Build history of the part. All positions in model axes, mm. A direction names the side the tool comes from. Round coordinates to 2 decimals unless told otherwise and drop trailing zeros. Order: outer loops, then holes, each group sorted by start corner. A loop starts at its lowest first (then second) coordinate and runs counter-clockwise, first axis right, second up. Notation, with made-up numbers: M -34,5 L 9,5 A12 cw 9,15 Z; hole C -5,0.5 d1. An arc over 180 degrees is marked long. One line per item, written item: value. Start each with the question number.
Item 1: Band-saw the part on A-A, the plane x = -9. Write the cut outline in (y, z).
Item 2: Probe L1, parallel to Y at x = 15, z = 0.3; L2, parallel to Y at x = 16.5, z = 0.4. List the from-to ranges inside material, lowest first.
Item 3: Two-plate mould, pull along X, no slides. Class faces 3 (the cylindrical face through (17.1, 10.86, 0.69)), 4 (the flat face through (17, 75, 1)), 5 (the flat face through (10, 74, 1)): +X half, -X half, draft (parallel to the pull), parting line (faces both ways), or undercut.
Item 4: Tool access for faces 1 (the flat face through (-7, 75, 1)), 2 (the flat face through (15, 73, 1)): list every direction of +Z, -Z, +X, -X, +Y, -Y with a clear straight run to the whole face (end or side of a thin tool).
```python
from build123d import *

# Parameters (mm, degrees)
F1_DEPTH = 1.4


with BuildPart() as f1:
    # F0 (on Top) → F1 (new body)
    with BuildSketch(Plane.XY):
        with BuildLine():
            Line((-18, 75), (-20, 75))
            Line((-20, 75), (-20, 73))
            Line((-20, 73), (-20, 13))
            ThreePointArc((-20, 13), (-19.12132, 10.87868), (-17, 10))
            Line((-17, 10), (-13, 10))
            Line((-13, 10), (13, 10))
            Line((13, 10), (15, 10))
            ThreePointArc((15, 10), (17.12132, 10.87868), (18, 13))
            Line((18, 13), (18, 73))
            Line((18, 73), (18, 75))
            Line((18, 75), (16, 75))
            Line((16, 75), (16, 73))
            Line((16, 73), (14, 73))
            Line((14, 73), (14, 75))
            Line((14, 75), (12, 75))
            Line((12, 75), (12, 73))
            Line((12, 73), (10, 73))
            Line((10, 73), (10, 75))
            Line((10, 75), (8, 75))
            Line((8, 75), (8, 73))
            Line((8, 73), (6, 73))
            Line((6, 73), (6, 75))
            Line((6, 75), (4, 75))
            Line((4, 75), (4, 73))
            Line((4, 73), (2, 73))
            Line((2, 73), (2, 75))
            Line((2, 75), (0, 75))
            Line((0, 75), (0, 73))
            Line((0, 73), (-2, 73))
            Line((-2, 73), (-2, 75))
            Line((-2, 75), (-4, 75))
            Line((-4, 75), (-4, 73))
            Line((-4, 73), (-6, 73))
            Line((-6, 73), (-6, 75))
            Line((-6, 75), (-8, 75))
            Line((-8, 75), (-8, 73))
            Line((-8, 73), (-10, 73))
            Line((-10, 73), (-10, 75))
            Line((-10, 75), (-12, 75))
            Line((-12, 75), (-12, 73))
            Line((-12, 73), (-14, 73))
            Line((-14, 73), (-14, 75))
            Line((-14, 75), (-16, 75))
            Line((-16, 75), (-16, 73))
            Line((-16, 73), (-18, 73))
            Line((-18, 73), (-18, 75))
        make_face()
    extrude(amount=F1_DEPTH)


solid = f1.part
```
Output:
1. outline: M 10,0 L 73,0 L 73,1.4 L 10,1.4 Z
2. L1: y = 10 to 73
2. L2: y = 10.4 to 75
3. face 3: +X half
3. face 4: draft
3. face 5: undercut
4. face 1: +Z, -Z, +X, -X, +Y
4. face 2: +Z, -Z, +Y
